Autodesk Inventor part; units mm, degrees
ref_plane "YZ Plane" through (0, 0, 0) normal (1, 0, 0) x (0, 1, 0)
ref_plane "XZ Plane" through (0, 0, 0) normal (0, 1, 0) x (-1, 0, 0)
ref_plane "XY Plane" through (0, 0, 0) normal (0, 0, 1) x (1, 0, 0)
sketch "スケッチ1" plane through (0, 0, 0) normal (0, 1, 0) x (-1, 0, 0)
  point P0 (0, 0)
sketch "スケッチ2" plane through (0, 0, 0) normal (0, 1, 0) x (-1, 0, 0)
  line L0 (0.845, -60.969) -> (0.845, -330.969)
  line L1 (0, 0) -> (0, -1.5537)
  line L2 (-202.155, -60.969) -> (-202.155, -330.969)
  arc A0 (-202.155, -330.969) -> (0.845, -330.969) centre (-100.655, -330.969) ccw
  line L3 (0.845, -60.969) -> (0.845, 309.031)
  line L4 (-202.155, -60.969) -> (-202.155, 309.031)
  arc A1 (0.845, 309.031) -> (-202.155, 309.031) centre (-100.655, 309.031) ccw
  dimension "d0" = 270
  dimension "d1" = 203
extrude "押し出し1" add sketch "スケッチ2" against normal blind 10
sketch "スケッチ4" plane through (0, -10, 0) normal (0, -1, 0) x (1, 0, 0)
  line L0 (73.655, -234.969) -> (127.655, -234.969)
  line L1 (127.655, -234.969) -> (127.655, -310.969)
  line L2 (127.655, -310.969) -> (73.655, -310.969)
  line L3 (73.655, -310.969) -> (73.655, -234.969)
  line L4 (202.155, -330.969) -> (202.155, 309.031)
  line L5 (-0.845, 309.031) -> (-0.845, -330.969)
  arc A0 (-0.845, -330.969) -> (202.155, -330.969) centre (100.655, -330.969) ccw
  line L6 (-0.845, -10.969) -> (202.155, -10.969)
  arc A1 (202.155, 309.031) -> (-0.845, 309.031) centre (100.655, 309.031) ccw
  line L7 (73.655, 213.031) -> (127.655, 213.031)
  line L8 (127.655, 213.031) -> (127.655, 289.031)
  line L9 (127.655, 289.031) -> (73.655, 289.031)
  line L10 (73.655, 289.031) -> (73.655, 213.031)
  circle A2 centre (79.655, -299.219) radius 2.75
  line L11 (100.655, -256.1001) -> (100.655, -272.969)
  circle A3 centre (79.655, -245.219) radius 2.75
  circle A4 centre (121.655, -299.219) radius 2.75
  circle A5 centre (121.655, -245.219) radius 2.75
  line L12 (73.655, 213.031) -> (127.655, 213.031)
  line L13 (127.655, 213.031) -> (127.655, 289.031)
  line L14 (127.655, 289.031) -> (73.655, 289.031)
  line L15 (73.655, 289.031) -> (73.655, 213.031)
  circle A6 centre (79.655, 277.281) radius 2.75
  line L16 (100.655, 234.1622) -> (100.655, 251.031)
  circle A7 centre (79.655, 223.281) radius 2.75
  circle A8 centre (121.655, 223.281) radius 2.75
  circle A9 centre (121.655, 277.281) radius 2.75
  point P0 (0, 0)
  dimension "d4" = 74.5
  dimension "d5" = 74.5
  dimension "d6" = 54
  dimension "d7" = 76
  dimension "d8" = 20
  dimension "d9" = 320
  dimension "d17" = 5.5
  dimension "d18" = 11.75
  dimension "d19" = 6
  dimension "d20" = 27
  dimension "d21" = 5.5
  dimension "d22" = 10.25
  dimension "d23" = 6
hole "穴2" at (79.655, -10, -245.219) at (79.655, -10, -299.219) at (121.655, -10, -299.219) at (121.655, -10, -245.219) direction (0, 1, 0) diameter 5.5 end through all
hole "穴3" at (79.655, -10, 223.281) at (121.655, -10, 223.281) at (121.655, -10, 277.281) at (79.655, -10, 277.281) direction (0, 1, 0) diameter 5.5 end through all
properties part number "sfp_smartboard_deck_upper" material "合板、仕上げ"
Source: CAD feature listing. Evaluate the final solid. Frame: model axes, mm. Give positions to 0.01 mm unless a question says otherwise; leave off trailing zeros. Write each loop counter-clockwise with the first axis right and the second up, starting at its lowest first coordinate (ties: lowest second). Pieces come first, ordered by that corner, then holes. Notation, with made-up numbers: M 80.5,-10.5 L 134.5,-10.5 A10 ccw 134.5,5.5 Z; hole C 33,-6.75 d6. An arc over 180 degrees is marked long. Answer as a JSON object with one key per item and string values.
Q1. Cut plane A-A, the plane y = -5. Count the separate pieces of the cut face and the enclosed holes in it, then the cut area to 3 significant figures.
Geometry check:
{"separate pieces": "1", "enclosed holes": "8", "area": "162,000 mm^2"}
Q2. Contact query for flat-ended pins moving along their axis: P1, Ø7, axis at x = 121.655, z = 277.281, coming from the +Y side; P2, Ø2, axis at x = 135.5, y = -1.5, coming from the -Z side; P3, Ø2, axis at x = 167.5, y = -6.5, coming from the +Z side; P4, Ø6, axis at x = 116, y = -3.5, coming from the +Z side. Output: stop coordinate, or through.
Geometry check:
{"P1": "stops at y = 0", "P2": "stops at z = -426.66", "P3": "stops at z = 386.28", "P4": "stops at z = 409.78"}
Q3. Cut plane C-C, the plane x = 169. Return the cut outline in (y, z), then the cut area to 3 significant figures.
Geometry check:
{"outline": "M -10,-406.01 L 0,-406.01 L 0,384.07 L -10,384.07 Z", "area": "7,900 mm^2"}
Q4. Mould query, pull axis Z, two halves, no side actions, for faces 1 (the face through (102.887, -4.93, -432.444)), 2 (the face through (102, 0, -5)), 3 (the face through (98.423, -4.93, 410.506)). Classes: +Z half, -Z half, draft (parallel to the pull), parting line (faces both ways), or undercut.
Geometry check:
{"face 1": "-Z half", "face 2": "draft", "face 3": "+Z half"}
Q5. Ray query, line 1 along Z through (x, y) = (98.5, -8.25); line 2 along Z through (x, y) = (77.5, -5.5); line 3 along Z through (x, y) = (105.5, -2.5). Return the intervals inside material, ascending.
Geometry check:
{"line 1": "z = -432.45 to 410.51", "line 2": "z = -429.79 to -300.93, -297.51 to -246.93, -243.51 to 221.57, 224.99 to 275.57, 278.99 to 407.85", "line 3": "z = -432.35 to 410.42"}
Q6. Cut plane B-B, the plane z = 359. Return the cut outline in (x, y), then the cut area to 3 significant figures.
Geometry check:
{"outline": "M 12.31,-10 L 189,-10 L 189,0 L 12.31,0 Z", "area": "1,770 mm^2"}
